Autodesk Inventor part; units mm, degrees
ref_plane "YZ Plane" through (0, 0, 0) normal (1, 0, 0) x (0, 1, 0)
ref_plane "XZ Plane" through (0, 0, 0) normal (0, 1, 0) x (-1, 0, 0)
ref_plane "XY Plane" through (0, 0, 0) normal (0, 0, 1) x (1, 0, 0)
sketch "Sketch1" plane through (0, 0, 0) normal (0, 0, 1) x (1, 0, 0)
  circle A0 centre (0, 0) radius 2.9
  dimension "d0" = 5.8
extrude "Extrusion1" add sketch "Sketch1" along normal blind 1.2
sketch "Sketch2" plane through (0, 0, 0) normal (0, 0, 1) x (1, 0, 0)
  circle A0 centre (0, 0) radius 2.9
  circle A1 centre (0, 0) radius 3.6
  dimension "d3" = 7.2
extrude "Extrusion2" add sketch "Sketch2" against normal blind 0.8 contours A0 | A1
sketch "Sketch3" plane through (0, 0, 1.2) normal (0, 0, 1) x (1, 0, 0)
  point P0 (0, 0)
hole "Hole1" at (0, 0, 1.2) direction (0, 0, -1) diameter 5 end through all
properties part number "LabyrinthSealInner"
Can you work these out from the model? Positions are in its coordinate system, mm. Give positions to 0.01 mm unless a question says otherwise; leave off trailing zeros. Order: outer loops, then holes, each group sorted by start corner. A loop starts at its lowest first (then second) coordinate and runs counter-clockwise, first axis right, second up. Notation, with made-up numbers: M -13.5,-22 L 10.5,-22 A26 ccw 10.5,1 Z; hole C 77,32.25 d3. An arc over 180 degrees is marked long. Use one line per item in the form item = value.
Item 1: If I drill on line 1 along Y through (x, z) = (0, 0.5); line 2 along X through (y, z) = (-1.5, 0.2); line 3 along Y through (x, z) = (2.25, 0.9), over which ranges is the centre line in solid material (lowest first)? Write a range as [from, to].
Values follow:
line_1 = [-2.9, -2.5], [2.5, 2.9]
line_2 = [-2.48, -2], [2, 2.48]
line_3 = [-1.83, -1.09], [1.09, 1.83]
Item 2: If we section it at A-A, the plane x = 0: Write out the boundary of the cut face in (y, z).
Values follow:
outline = M -3.6,-0.8 L -2.5,-0.8 L -2.5,1.2 L -2.9,1.2 L -2.9,0 L -3.6,0 Z; M 2.5,-0.8 L 3.6,-0.8 L 3.6,0 L 2.9,0 L 2.9,1.2 L 2.5,1.2 Z
Item 3: If we section it at C-C, the plane z = -0.2: Write out the boundary of the cut face in (x, y).
Values follow:
outline = C 0,0 d7.2; hole C 0,0 d5
Item 4: Thinking about a two-plate mould opening in X: for faces 1 (the cylindrical face through (3.434, 1.081, -0.394)), 2 (the cylindrical face through (2.44, 0.54, 0.19)), 3 (the flat face through (-0.9, 2.5, -0.8)), which applies, pulls with the +X half, pulls with the -X half, needs draft (parallel to the pull), parting line crosses it, or undercut?
Values follow:
face_1 = parting line crosses it
face_2 = undercut
face_3 = needs draft
Item 5: Will this pin go through, and if not, where does the flat tip stop? pin 1 Ø4 at (x, y) = (0, 0) entering from -Z.
Values follow:
pin_1 = through
Item 6: If we section it at D-D, the plane x = 2.75: Write out the boundary of the cut face in (y, z), and give its area (3 significant figures).
Values follow:
outline = M -2.32,-0.8 L 2.32,-0.8 L 2.32,0 L 0.92,0 L 0.92,1.2 L -0.92,1.2 L -0.92,0 L -2.32,0 Z
area = 5.93 mm^2
